from build123d import *

# Parameters (mm, degrees)
SKETCH2_R            = 41.91
SKETCH2_R_2          = 38.1
BASE_CYLINDER_DEPTH  = 292.1
SKETCH3_R            = 63.5
SKETCH3_R_2          = 38.1
AFT_FLANGE_DEPTH     = 12.7
SKETCH4_R            = 63.5
SKETCH4_R_2          = 38.1
FORWARD_FLANGE_DEPTH = 12.7


with BuildPart() as part:
    # Sketch2 → Base Cylinder (new body)
    with BuildSketch(Plane(origin=(0, 0, 0), x_dir=(1, 0, 0), z_dir=(0, 1, 0))):
        Circle(SKETCH2_R)
        Circle(SKETCH2_R_2, mode=Mode.SUBTRACT)
    extrude(amount=BASE_CYLINDER_DEPTH)

    # Sketch3 → Aft Flange (add)
    with BuildSketch(Plane.XZ):
        Circle(SKETCH3_R)
        Circle(SKETCH3_R_2, mode=Mode.SUBTRACT)
    extrude(amount=-AFT_FLANGE_DEPTH)

    # Sketch4 → Forward Flange (add)
    with BuildSketch(Plane(origin=(0, 292.1, 0), x_dir=(1, 0, 0), z_dir=(0, 1, 0))):
        Circle(SKETCH4_R)
        Circle(SKETCH4_R_2, mode=Mode.SUBTRACT)
    extrude(amount=-FORWARD_FLANGE_DEPTH)


solid = part.part
The model under review builds one solid part; all positions refer to its coordinate system, in mm. A direction names the side the tool comes from. Coordinates: 2 decimals unless noted, no trailing zeros. Write each loop counter-clockwise with the first axis right and the second up, starting at its lowest first coordinate (ties: lowest second). Pieces come first, ordered by that corner, then holes. Notation, with made-up numbers: (-33, 18.25) - (-17, 18.25) arc R14 cw to (-17, 44.25) - close; hole circle Ø9 at (73.25, -34). An arc over 180 degrees is marked (long way). Answer as CSV lines item,"result".
(1) Clearance check with flat-ended pins moving along their axes: pin 1 Ø6 at (y, z) = (40.5, 22.5) entering from +X; pin 2 Ø4 at (y, z) = (111.5, -17) entering from +X; pin 3 Ø6 at (y, z) = (161, -6) entering from +X. State where each tip first meets the part, or that it passes through.
Data:
pin 1,"stops at x = 37.1"
pin 2,"stops at x = 39.13"
pin 3,"stops at x = 41.8"
(2) Tool access review of faces 1 (the flat face through (27.3, 292.1, 27.3)), 2 (the flat face through (41, 12.7, -13)): name each direction out of +Z, -Z, +X, -X, +Y, -Y from which nothing blocks a thin tool from reaching the whole face with its end or side.
Data:
face 1,"+Z, -Z, +X, -X, +Y"
face 2,"none"
(3) We need section A-A (x = 0). Give the boundary of the cut face in (y, z).
Data:
outline,"(0, -63.5) - (12.7, -63.5) - (12.7, -41.91) - (279.4, -41.91) - (279.4, -63.5) - (292.1, -63.5) - (292.1, -38.1) - (0, -38.1) - close; (0, 38.1) - (292.1, 38.1) - (292.1, 63.5) - (279.4, 63.5) - (279.4, 41.91) - (12.7, 41.91) - (12.7, 63.5) - (0, 63.5) - close"
(4) We need section C-C (y = 69.5). Give the boundary of the cut face in (x, z), plus the area to 3 significant figures.
Data:
outline,"circle Ø83.82 at (0, 0); hole circle Ø76.2 at (0, 0)"
area,"958 mm2"
(5) We need section D-D (x = 45.5). Give the boundary of the cut face in (y, z).
Data:
outline,"(0, -44.29) - (12.7, -44.29) - (12.7, 44.29) - (0, 44.29) - close; (279.4, -44.29) - (292.1, -44.29) - (292.1, 44.29) - (279.4, 44.29) - close"
(6) Mouldability with a two-part tool opening along Y and no side actions: class faces 3 (the cylindrical face through (-13.77, 6.26, -61.99)), 4 (the cylindrical face through (-5.456, 144.183, -41.553)), 5 (the flat face through (27.3, 0, -27.3)) as pulls with the +Y half, pulls with the -Y half, needs draft (parallel to the pull), parting line crosses it, or undercut.
Data:
face 3,"needs draft"
face 4,"undercut"
face 5,"pulls with the -Y half"
(7) We need section B-B (z = 0). Give the boundary of the cut face in (x, y).
Data:
outline,"(-63.5, 0) - (-38.1, 0) - (-38.1, 292.1) - (-63.5, 292.1) - (-63.5, 279.4) - (-41.91, 279.4) - (-41.91, 12.7) - (-63.5, 12.7) - close; (38.1, 0) - (63.5, 0) - (63.5, 12.7) - (41.91, 12.7) - (41.91, 279.4) - (63.5, 279.4) - (63.5, 292.1) - (38.1, 292.1) - close"
(8) For line 1 along Z through (x, y) = (0, 72); line 2 along Y through (x, z) = (-38.5, -19.5); line 3 along Z through (x, y) = (20, 145), list the stretches that pass through material, from the lowest coordinate up. Write a range as [from, to].
Data:
line 1,"z = [-41.91, -38.1], [38.1, 41.91]"
line 2,"y = [0, 12.7], [279.4, 292.1]"
line 3,"z = [-36.83, -32.43], [32.43, 36.83]"
